```python
from build123d import *

# Parameters (mm, degrees)
SUSP_FR_TIE_ROD_PROFILE_R             = 8
SUSP_FR_TIE_ROD_ROD_END_IN_PROFILE_R  = 11
SUSP_FR_TIE_ROD_ROD_END_OUT_PROFILE_R = 11


with BuildPart() as part:
    # SUSP_FR_tie_rod: sweep along a curve in space
    with BuildLine() as susp_fr_tie_rod_path:
        Line((270, -90.4, -82.3915), (590.293517, -204.990503, -103.750386))
    # SUSP_FR_tie_rod profile (on start of the path) → SUSP_FR_tie_rod (sweep)
    with BuildSketch(Plane(origin=(270, -90.4, -82.3915), x_dir=(0.33685766905299525, 0.9415555803032463, 0), z_dir=(0.9397050891891743, -0.3361956240964046, -0.06266456487038859))):
        Circle(SUSP_FR_TIE_ROD_PROFILE_R)
    sweep(path=susp_fr_tie_rod_path.line)

    # SUSP_FR_tie_rod_rod_end_in: sweep along a curve in space
    with BuildLine() as susp_fr_tie_rod_rod_end_in_path:
        Line((271.21105, -91.0008904, -75.5232915), (268.78895, -89.7991096, -89.2597085))
    # SUSP_FR_tie_rod_rod_end_in profile (on start of the path) → SUSP_FR_tie_rod_rod_end_in (sweep)
    with BuildSketch(Plane(origin=(271.21105, -91.0008904, -75.5232915), x_dir=(-0.9848077644799927, 0, 0.17364811262987942), z_dir=(-0.17300714396088532, 0.08584148626193362, -0.9811726491167799))):
        Circle(SUSP_FR_TIE_ROD_ROD_END_IN_PROFILE_R)
    sweep(path=susp_fr_tie_rod_rod_end_in_path.line)

    # SUSP_FR_tie_rod_rod_end_out: sweep along a curve in space
    with BuildLine() as susp_fr_tie_rod_rod_end_out_path:
        Line((591.504567, -205.591393, -96.882177), (589.082466, -204.389612, -110.618594))
    # SUSP_FR_tie_rod_rod_end_out profile (on start of the path) → SUSP_FR_tie_rod_rod_end_out (sweep)
    with BuildSketch(Plane(origin=(591.504567, -205.591393, -96.882177), x_dir=(-0.9848077522197362, 0, 0.17364818216126232), z_dir=(-0.17300721303932562, 0.08584149938158056, -0.9811726357885688))):
        Circle(SUSP_FR_TIE_ROD_ROD_END_OUT_PROFILE_R)
    sweep(path=susp_fr_tie_rod_rod_end_out_path.line)


solid = part.part
```
Model file for the job. Use its own axes, mm. A direction names the side the tool comes from. Coordinates: 2 decimals unless noted, no trailing zeros. Write item = value, one per line. Start each with the question number.
Item 1: 3-axis set-ups, long thin cutter, end or side, ignore diameter. For faces 1 (the face through (591.725, -204.236, -111.071)), 2 (the face through (598.773, -211.651, -105.928)), 3 (the face through (268.9, -90.8, -75.1)): which of +Z, -Z, +X, -X, +Y, -Y reach the whole face in a straight line?
Item 2: Drop flat-ended pins along their axis: pin 1 Ø4 at (x, z) = (341, -84) entering from -Y; pin 2 Ø5 at (x, z) = (441, -95) entering from -Y; pin 3 Ø8 at (x, z) = (315.5, -84.5) entering from +Y. Give the stop position or say it passes through.
Item 3: Wall check: probe 1 along Y at (x, z) = (413.5, -85); probe 2 along Y at (x, z) = (389, -84); probe 3 along Z at (x, y) = (528.5, -180.5). Give the ranges that are in metal, low to high. Write a range as [from, to].
Answers:
q1.face_1 = -Z
q1.face_2 = none
q1.face_3 = +Z
q2.pin_1 = -124.54
q2.pin_2 = -160.94
q2.pin_3 = -96.76
q3.probe_1 = [-145.79, -137.36]
q3.probe_2 = [-138.04, -127.61]
q3.probe_3 = [-107.27, -91.89]
